The listing builds one solid part. Answer for the finished solid, in the listing's coordinates (mm). A direction names the side the tool comes from. Give positions to 0.01 mm unless a question says otherwise; leave off trailing zeros. Write each loop counter-clockwise with the first axis right and the second up, starting at its lowest first coordinate (ties: lowest second). Pieces come first, ordered by that corner, then holes. Notation, with made-up numbers: M 87.25,58 L 131.25,58 A9 cw 131.25,62 Z; hole C 33.25,74 d8. An arc over 180 degrees is marked long. Answer as a JSON object with one key per item and string values.
```python
from build123d import *

# Parameters (mm, degrees)
SKETCH_W        = 33.2
SKETCH_H        = 7
SKETCH_R        = 1.6
PAD_DEPTH       = 25
SKETCH001_R     = 1.6
PAD001_DEPTH    = 33.2
SKETCH002_W     = 7.5
SKETCH002_H     = 10
SKETCH002_W_2   = 3
POCKET_DEPTH    = 25.001
FILLET_R        = 2.99
FILLET001_R     = 4.99
POCKET001_DEPTH = 2.5


with BuildPart() as part:
    # Sketch → Pad (new body)
    with BuildSketch(Plane.XY):
        Rectangle(SKETCH_W, SKETCH_H)
        with Locations((-13, 0)):
            Circle(SKETCH_R, mode=Mode.SUBTRACT)
        with Locations((13, 0)):
            Circle(SKETCH_R, mode=Mode.SUBTRACT)
    extrude(amount=PAD_DEPTH)

    # Sketch001 (on Face4 of Pad) → Pad001 (join)
    with BuildSketch(Plane(origin=(-16.6, 0, 0), x_dir=(0, -1, 0), z_dir=(-1, 0, 0))):
        with BuildLine():
            Line((-3.5, 17.5), (-3.5, 7.5))
            Line((-8.5, 7.5), (-3.5, 7.5))
            ThreePointArc((-8.5, 17.5), (-13.5, 12.5), (-8.5, 7.5))
            Line((-3.5, 17.5), (-8.5, 17.5))
        make_face()
        with Locations((-8.5, 12.5)):
            Circle(SKETCH001_R, mode=Mode.SUBTRACT)
    extrude(amount=-PAD001_DEPTH)

    # Sketch002 (on Face11 of Pad001) → Pocket (cut, through all)
    with BuildSketch(Plane.XY.offset(25)):
        with Locations((0, 8.5)):
            Rectangle(SKETCH002_W, SKETCH002_H)
        with Locations((-15.1, 8.5)):
            Rectangle(SKETCH002_W_2, SKETCH002_H)
        with Locations((15.1, 8.5)):
            Rectangle(SKETCH002_W_2, SKETCH002_H)
    extrude(amount=-POCKET_DEPTH, mode=Mode.SUBTRACT)

    # Fillet
    fillet_edges = [part.edges().sort_by_distance(p)[0] for p in [
        (-16.6, 3.5, 12.5),
        (-16.6, -3.5, 12.5),
        (16.6, -3.5, 12.5),
        (16.6, 3.5, 12.5),
    ]]
    fillet(fillet_edges, radius=FILLET_R)

    # Fillet001
    fillet001_edges = [part.edges().sort_by_distance(p)[0] for p in [
        (8.675, 3.5, 17.5),
        (-8.675, 3.5, 17.5),
        (8.675, 3.5, 7.5),
        (-8.675, 3.5, 7.5),
    ]]
    fillet(fillet001_edges, radius=FILLET001_R)

    # Sketch003 (on Face2 of Fillet001) → Pocket001 (cut)
    with BuildSketch(Plane(origin=(-13.6, 0, 0), x_dir=(0, -1, 0), z_dir=(-1, 0, 0))):
        Polygon((-5.266838, 12.5), (-6.883419, 15.3), (-10.116581, 15.3), (-11.733162, 12.5), (-10.116581, 9.7), (-6.883419, 9.7), align=None)
    extrude(amount=-POCKET001_DEPTH, mode=Mode.SUBTRACT)


solid = part.part
```
1. A cutting plane is placed at A-A, the plane x = -13. Count the separate pieces of the cut face and the enclosed holes in it, plus the area to 3 significant figures.
Verdict:
{"separate pieces": "2", "enclosed holes": "1", "area": "168 mm2"}
2. Flat-ended cylindrical pins translate along their axes: pin 1 (6 mm diameter, centred on y = 1, z = 14, fed in from +X); pin 2 (7.5 mm diameter, centred on x = 3, z = 17, fed in from +Y); pin 3 (4 mm diameter, centred on y = 8.5, z = 12.5, fed in from +X); pin 4 (4.5 mm diameter, centred on y = 7.5, z = 12.5, fed in from -X). Find the tip coordinate at first contact, or state that the pin passes through.
Verdict:
{"pin 1": "stops at x = 16.6", "pin 2": "stops at y = 13.43", "pin 3": "stops at x = 13.6", "pin 4": "stops at x = -13.6"}
3. For faces 1 (the flat face through (3.75, 6, 13)), 2 (the flat face through (13.6, 6, 13)), 3 (the cylindrical face through (-15.75, 2.6, 12.32)), 4 (the flat face through (0, 3.5, 12)), 5 (the flat face through (-12.368, 6.086, 11.08)), determine the directions among +Z, -Z, +X, -X, +Y, -Y from which every point of the face is accessible in a straight line to the end or side of a thin tool.
Verdict:
{"face 1": "+Z, -Z, +Y", "face 2": "+Z, -Z, +X, +Y", "face 3": "+Z, -Z, -X, +Y", "face 4": "+Y", "face 5": "-X"}
4. A cutting plane is placed at D-D, the plane y = 11. Give the vertices of the cut face in (x, z), plus the area to 3 significant figures.
Verdict:
{"outline": "M -13.6,8.17 L -3.75,8.17 L -3.75,16.83 L -13.6,16.83 L -13.6,13.77 L -11.1,13.77 L -11.1,11.23 L -13.6,11.23 Z; M 3.75,8.17 L 13.6,8.17 L 13.6,16.83 L 3.75,16.83 Z", "area": "164 mm2"}
5. Consider line 1 along X through (y, z) = (-1.25, 18.5); line 2 along Z through (x, y) = (11.25, 8.5); line 3 along Z through (x, y) = (-12.5, 8.75). Determine where each line is inside the solid, lowest interval first.
Verdict:
{"line 1": "x = -16.51 to -14, -12 to 12, 14 to 16.51", "line 2": "z = 7.5 to 10.9, 14.1 to 17.5", "line 3": "z = 7.51 to 9.7, 15.3 to 17.49"}
6. A cutting plane is placed at B-B, the plane y = 0. Give the vertices of the cut face in (x, z).
Verdict:
{"outline": "M -16.6,0 L -14.6,0 L -14.6,25 L -16.6,25 Z; M -11.4,0 L 11.4,0 L 11.4,25 L -11.4,25 Z; M 14.6,0 L 16.6,0 L 16.6,25 L 14.6,25 Z"}
7. The mould has two halves that part along X. Classify faces 6 (the cylindrical face through (-8.606, 4.923, 19.001)), 7 (the cylindrical face through (11.4, 0.07, 12.32)), 8 (the cylindrical face through (-15.75, -2.6, 12.68)): released by +X, released by -X, zero draft, split by the parting line, or undercut.
Verdict:
{"face 6": "zero draft", "face 7": "undercut", "face 8": "released by -X"}
